Geometry: final body of the model. Coordinates: model frame, mm. A direction names the side the tool comes from. Round coordinates to 2 decimals unless told otherwise and drop trailing zeros. Loops run counter-clockwise (first coordinate to the right, second up) from the corner with the lowest first, then second, coordinate; pieces in that order, holes last. Notation, with made-up numbers: (40, 57) - (55, 57) arc R15 ccw to (55, 62) - close; hole circle Ø4 at (66.25, 25). An arc over 180 degrees is marked (long way). Write item = value, one per line. Start each with the question number.
Item 1: First-contact query: pin 1 (1.5 mm diameter, centred on y = -0.5, z = 0.5, fed in from +X); pin 2 (1.5 mm diameter, centred on x = 3.5, y = 1.5, fed in from +Z). Flat tips, straight axial feed; report the tip coordinate or a pass-through.
Item 2: Section B-B (x = 1). Return loops of the section in (y, z), plus the area to 3 significant figures.
Item 3: Access query for faces 1 (the flat face through (1, 3, 0)), 2 (the cylindrical face through (2.6, -2, 2.2)). Directions: +Z, -Z, +X, -X, +Y, -Y. A direction counts if a zero-diameter tool reaches every point of the face in a straight line with its end or side. Return the directions, or none.
Item 4: Line query: line 1 (Z direction, x = 3.3, y = 0) (1 decimal); line 2 (Y direction, x = 3.9, z = 0). Output: solid intervals per line, ascending. Write a range as from..to.
Item 5: Draft query along Y for faces 3 (the cylindrical face through (0.99, 0.976, -0.748)), 4 (the flat face through (1, 1.5, 2.6)), 5 (the flat face through (1, -1.5, 2.6)), 6 (the cylindrical face through (2.848, 0.748, 0.976)). Return one class per face: pulls with the +Y half, pulls with the -Y half, needs draft (parallel to the pull), parting line crosses it, or undercut.
Autodesk Inventor part; units mm, degrees
ref_plane "YZ Plane" through (0, 0, 0) normal (1, 0, 0) x (0, 1, 0)
ref_plane "XZ Plane" through (0, 0, 0) normal (0, 1, 0) x (-1, 0, 0)
ref_plane "XY Plane" through (0, 0, 0) normal (0, 0, 1) x (1, 0, 0)
sketch "Sketch_1" plane through (0, 0, 0) normal (1, 0, 0) x (0, -1, 0)
  line L0 (-3, -1.7321) -> (0, -3.4641)
  line L1 (0, -3.4641) -> (3, -1.7321)
  line L2 (3, -1.7321) -> (3, 1.7321)
  line L3 (3, 1.7321) -> (0, 3.4641)
  line L4 (0, 3.4641) -> (-3, 1.7321)
  line L5 (-3, 1.7321) -> (-3, -1.7321)
extrude "Extrusion1" add sketch "Sketch_1" along normal blind 2
sketch "Sketch_2" plane through (0, 0, 0) normal (0, -1, 0) x (0, 0, -1)
  line L0 (0, -50) -> (0, 50)
  line L1 (2.3, 0) -> (6, 0)
  line L2 (6, 0) -> (6, 0.9914)
  line L3 (6, 0.9914) -> (2.3, 0)
revolve "Revolution1" cut sketch "Sketch_2" angle 360 about axis through (-50, 0, 0) along (-1, 0, 0)
sketch "Sketch_3" plane through (0, 0, 0) normal (0, -1, 0) x (0, 0, -1)
  line L0 (0, -50) -> (0, 50)
  line L1 (2.3, 2) -> (6, 1.0086)
  line L2 (6, 1.0086) -> (6, 2)
  line L3 (6, 2) -> (2.3, 2)
revolve "Revolution2" cut sketch "Sketch_3" angle 360 about axis through (-50, 0, 0) along (-1, 0, 0)
sketch "Sketch_4" plane through (0, 0, 0) normal (0, -1, 0) x (0, 0, -1)
  line L0 (0, -200) -> (0, 200)
  line L1 (0, 4) -> (2.38, 4)
  arc A0 (2.975, 3.405) -> (2.38, 4) centre (2.38, 3.405) ccw
  line L2 (2.975, 3.405) -> (2.975, 1.7543)
  line L3 (2.975, 1.7543) -> (0, 1.7543)
  line L4 (0, 1.7543) -> (0, 4)
revolve "Revolution3" add sketch "Sketch_4" angle 360 about axis through (-200, 0, 0) along (-1, 0, 0)
sketch "Sketch_5" plane through (0, 0, 0) normal (0, 0, 1) x (0, -1, 0)
  line L0 (0, -200) -> (0, 200)
  line L1 (0, 2) -> (1.5, 2)
  line L2 (1.5, 2) -> (1.2295, 1.7295)
  line L3 (1.2295, 1.7295) -> (1.2295, 0.2705)
  line L4 (1.2295, 0.2705) -> (1.5, 0)
  line L5 (1.5, 0) -> (0, 0)
  line L6 (0, 0) -> (0, 2)
revolve "Revolution4" cut sketch "Sketch_5" angle 360 about axis through (-200, 0, 0) along (-1, 0, 0)
thread "Thread1"
sketch "Sketch6" plane through (4, 0, 0) normal (1, 0, 0) x (0, 0, -1)
  point P0 (0, 0)
hole "Hole1" at (4, 0, 0) direction (-1, 0, 0) diameter 2.459 depth 2 counterbore diameter 3 counterbore depth 0.28
properties part number "652203A2"
Taken from the geometry:
q1.pin_1 = 3.72
q1.pin_2 = 2.88
q2.outline = (-3, -1.73) - (0, -3.46) - (3, -1.73) - (3, 1.73) - (0, 3.46) - (-3, 1.73) - close; hole circle Ø2.46 at (0, 0)
q2.area = 26.4 mm^2
q3.face_1 = +Z, -Z, +X, -X, +Y
q3.face_2 = +X
q4.line_1 = -3..-1.2, 1.2..3
q4.line_2 = -2.71..-1.5, 1.5..2.71
q5.face_3 = undercut
q5.face_4 = pulls with the +Y half
q5.face_5 = pulls with the -Y half
q5.face_6 = undercut
